Input: part model. Units: mm. Frame: model coordinates. Face numbers are marked on the shaded views. A direction names the side the tool comes from. Give positions to 0.01 mm unless a question says otherwise; leave off trailing zeros. Loops run counter-clockwise (first coordinate to the right, second up) from the corner with the lowest first, then second, coordinate; pieces in that order, holes last.
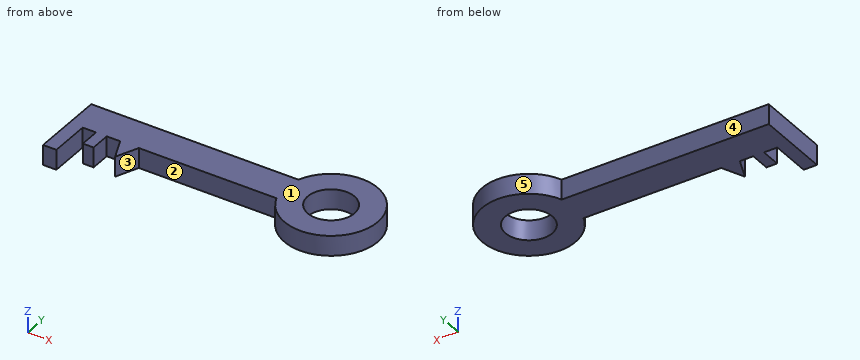
from build123d import *

# Parameters (mm, degrees)
F0_R     = 17.5
F0_W     = 10
F0_H     = 30
F0_W_2   = 8
F0_H_2   = 15
F1_DEPTH = 15


with BuildPart() as f1:
    # F0 (on Top) → F1 (new body)
    with BuildSketch(Plane.XY):
        Polygon((49.769913, 41.319751), (-105.230087, 41.319751), (-105.230087, 16.319751), (-95.230087, 16.319751), (-85.230087, 16.319751), (-77.230087, 16.319751), (-67.230087, 16.319751), (-53.230087, 16.319751), (49.769913, 16.319751), align=None)
        with BuildLine():
            ThreePointArc((49.769913, 16.319751), (117.461655, 28.819751), (49.769913, 41.319751))
            Line((49.769913, 41.319751), (49.769913, 16.319751))
        make_face()
        with Locations((82.461655, 28.819751)):
            Circle(F0_R, mode=Mode.SUBTRACT)
        with Locations((-100.230087, 1.319751)):
            Rectangle(F0_W, F0_H)
        Polygon((-60.230087, 0), (-53.230087, 16.319751), (-67.230087, 16.319751), align=None)
        with Locations((-81.230087, 8.819751)):
            Rectangle(F0_W_2, F0_H_2)
    extrude(amount=F1_DEPTH)


solid = f1.part
(1) Reachability of the marked faces 1 and 2 from +Z, -Z, +X, -X, +Y, -Y: full face, straight path, thin tool, end or side. Return the list, or none.
Values follow:
face 1: +Z, +X, -X, +Y, -Y
face 2: +Z, -Z, -Y
(2) Cut plane C-C (y = 5.5). Return the cut outline in (x, z).
Values follow:
outline: (-105.23, 0) - (-95.23, 0) - (-95.23, 15) - (-105.23, 15) - close; (-85.23, 0) - (-77.23, 0) - (-77.23, 15) - (-85.23, 15) - close; (-62.59, 0) - (-57.87, 0) - (-57.87, 15) - (-62.59, 15) - close; (56.36, 0) - (108.56, 0) - (108.56, 15) - (56.36, 15) - close
(3) Pin query (flat end, axial travel): pin 1 Ø2 at (x, y) = (-65, 25.5) entering from -Z; pin 2 Ø1.5 at (x, z) = (73.5, 9.5) entering from +Y; pin 3 Ø7.5 at (x, z) = (2, 9.5) entering from +Y; pin 4 Ø4 at (x, z) = (-0.5, 13) entering from -Y. Return the tip coordinate at first contact, or that it passes through.
Values follow:
pin 1: stops at z = 0
pin 2: stops at y = 62.84
pin 3: stops at y = 41.32
pin 4: stops at y = 16.32
(4) Mould query, pull axis X, two halves, no side actions, for the marked faces 3, 4 and 5. Classes: +X half, -X half, draft (parallel to the pull), parting line (faces both ways), or undercut.
Values follow:
face 3: undercut
face 4: draft
face 5: undercut
(5) Cut plane D-D (z = 12). Return the cut outline in (x, y), and give its area (3 significant figures).
Values follow:
outline: (-105.23, -13.68) - (-95.23, -13.68) - (-95.23, 16.32) - (-85.23, 16.32) - (-85.23, 1.32) - (-77.23, 1.32) - (-77.23, 16.32) - (-67.23, 16.32) - (-60.23, 0) - (-53.23, 16.32) - (49.77, 16.32) arc R35 ccw (long way) to (49.77, 41.32) - (-105.23, 41.32) - close; hole circle Ø35 at (82.46, 28.82)
area: 7,260 mm2
(6) Cut plane B-B (y = 21.5). Return the cut outline in (x, z).
Values follow:
outline: (-105.23, 0) - (66.57, 0) - (66.57, 15) - (-105.23, 15) - close; (98.36, 0) - (116.69, 0) - (116.69, 15) - (98.36, 15) - close
(7) Cut plane A-A (x = 78.5). Return the cut outline in (y, z), and give its area (3 significant figures).
Values follow:
outline: (-5.96, 0) - (11.77, 0) - (11.77, 15) - (-5.96, 15) - close; (45.87, 0) - (63.59, 0) - (63.59, 15) - (45.87, 15) - close
area: 532 mm2
(8) Ray query, probe 1 along X at (y, z) = (29.5, 8); probe 2 along X at (y, z) = (4, 5.5); probe 3 along X at (y, z) = (6, 14). Return the intervals inside material, ascending.
Values follow:
probe 1: x = -105.23 to 64.97, 99.95 to 117.46
probe 2: x = -105.23 to -95.23, -85.23 to -77.23, -61.95 to -58.51, 57.78 to 107.14
probe 3: x = -105.23 to -95.23, -85.23 to -77.23, -62.8 to -57.66, 55.92 to 109
